Can you work these out from the model? Positions are in its coordinate system, mm. Give positions to 0.01 mm unless a question says otherwise; leave off trailing zeros. Loops run counter-clockwise (first coordinate to the right, second up) from the corner with the lowest first, then second, coordinate; pieces in that order, holes last. Notation, with made-up numbers: (-11, -13) - (4, -13) arc R12 cw to (4, 7) - close; hole circle Ø6 at (-36.5, 61.5). An arc over 180 degrees is marked (long way). Answer as a JSON object with one key per item and string values.
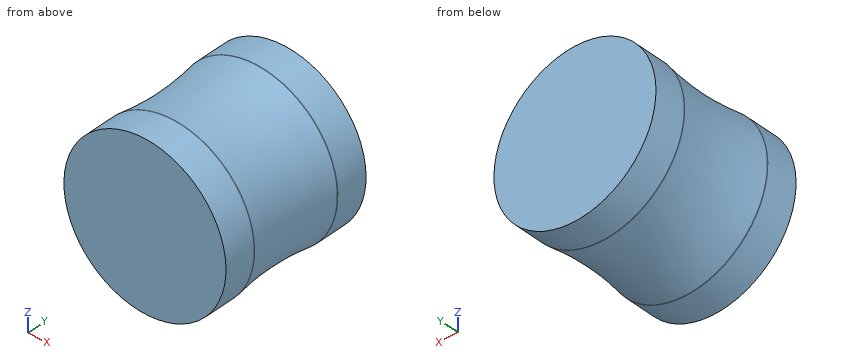
```python
from build123d import *


with BuildPart() as part:
    # Skizze1 → Rotation1 (revolve)
    with BuildSketch(Plane.XY, mode=Mode.PRIVATE) as rotation1_sk:
        with BuildLine():
            Line((109.527295839, -62.872686635), (109.527295839, -105.259657321))
            Line((109.527295839, -105.259657321), (0, -105.259657321))
            Line((0, -105.259657321), (0, 105.259657321))
            Line((0, 105.259657321), (109.527295839, 105.259657321))
            Line((109.527295839, 105.259657321), (109.527295839, 62.872686635))
            ThreePointArc((109.527295839, 62.872686635), (109.511559563, 62.47630913), (109.464449789, 62.082426628))
            ThreePointArc((109.464449789, 62.082426628), (104.527295839, 0), (109.464449789, -62.082426628))
            ThreePointArc((109.464449789, -62.082426628), (109.511559563, -62.47630913), (109.527295839, -62.872686635))
        make_face()
    revolve(rotation1_sk.sketch.rotate(Axis((0, 105.259657321, 0), (0, -1, 0)), 90), axis=Axis((0, 105.259657321, 0), (0, -1, 0)))  # turned: the seam where the file's is


solid = part.part
```
1) Imagine slicing it at A-A on z = 0. Write out the boundary of the cut face in (x, y), and give its area (3 significant figures).
Check sheet entries:
{"outline": "(-109.53, -105.26) - (109.53, -105.26) - (109.53, -62.87) arc R5 ccw to (109.46, -62.08) arc R392.8 cw to (109.46, 62.08) arc R5 ccw to (109.53, 62.87) - (109.53, 105.26) - (-109.53, 105.26) - (-109.53, 62.87) arc R5 ccw to (-109.46, 62.08) arc R392.8 cw to (-109.46, -62.08) arc R5 ccw to (-109.53, -62.87) - close", "area": "45,300 mm2"}
2) Imagine slicing it at B-B on x = 0. Write out the boundary of the cut face in (y, z), and give its area (3 significant figures).
Check sheet entries:
{"outline": "(-105.26, -109.53) - (-62.87, -109.53) arc R5 ccw to (-62.08, -109.46) arc R392.8 cw to (62.08, -109.46) arc R5 ccw to (62.87, -109.53) - (105.26, -109.53) - (105.26, 109.53) - (62.87, 109.53) arc R5 ccw to (62.08, 109.46) arc R392.8 cw to (-62.08, 109.46) arc R5 ccw to (-62.87, 109.53) - (-105.26, 109.53) - close", "area": "45,300 mm2"}
3) I'm going to push flat-ended pins straight in: P1, Ø12, axis at x = -51, y = -9, coming from the +Z side; P2, Ø4, axis at y = 61, z = 82.5, coming from the +X side; P3, Ø1, axis at x = -37, y = 45, coming from the +Z side. Where does each tip first touch, or does it pass through?
Check sheet entries:
{"P1": "z = 94.46", "P2": "x = 73.97", "P3": "z = 100.71"}
4) Imagine slicing it at C-C on y = 38.5. Write out the boundary of the cut face in (x, z), and give its area (3 significant figures).
Check sheet entries:
{"outline": "circle Ø212.84 at (0, 0)", "area": "35,600 mm2"}
5) Imagine slicing it at D-D on y = -12. Write out the boundary of the cut face in (x, z).
Check sheet entries:
{"outline": "circle Ø209.42 at (0, 0)"}
6) I need wall thicknesses on L1, parallel to X at y = -19, z = -6.5; L2, parallel to X at y = -77.5, z = 95.5; L3, parallel to Z at x = 76, y = -58.5. Which ranges of each line are inside material? Lowest first, please.
Check sheet entries:
{"L1": "-104.79 to 104.79", "L2": "-53.63 to 53.63", "L3": "-78.01 to 78.01"}
